Could you check a few things on this model? Use its own coordinates, in mm. Face numbers are marked on the shaded views. A direction names the side the tool comes from. Round coordinates to 2 decimals unless told otherwise and drop trailing zeros. Loops run counter-clockwise (first coordinate to the right, second up) from the corner with the lowest first, then second, coordinate; pieces in that order, holes last.
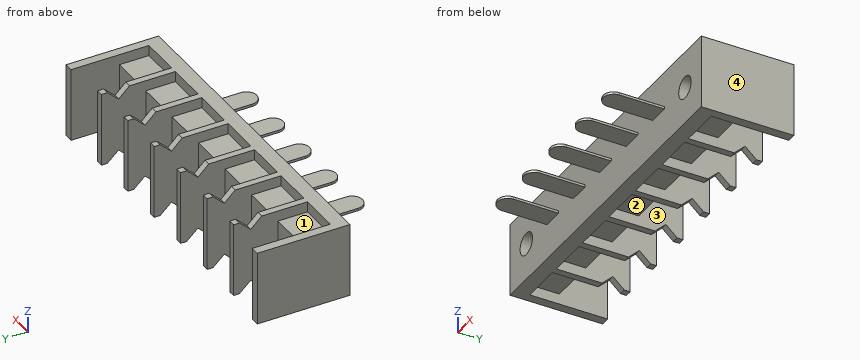
from build123d import *

# Parameters (mm, degrees)
SKETCH_1_W          = 69.1
SKETCH_1_H          = 15
EXTRUDE_1_DEPTH     = 18.8
SKETCH_2_W          = 65.5
SKETCH_2_H          = 15
CUT_EXTRUDE_1_DEPTH = 0.8
SKETCH_4_W          = 8.2
SKETCH_4_H          = 15
CUT_EXTRUDE_2_DEPTH = 9
SKETCH_5_W          = 8.2
SKETCH_5_H          = 2.132429546
CUT_EXTRUDE_3_DEPTH = 15
SKETCH_6_W          = 4.2
SKETCH_6_H          = 0.5
EXTRUDE_2_DEPTH     = 11.2
SKETCH_7_R          = 2.25
CUT_EXTRUDE_4_DEPTH = 41.718454047
CUT_EXTRUDE_START   = -49.1
CUT_EXTRUDE_5_DEPTH = 49.1
FILLET_1_R          = 2.1


with BuildPart() as part:
    # 草图1 → 拉伸1 (new body)
    with BuildSketch(Plane(origin=(0, 0, 0), x_dir=(1, 0, 0), z_dir=(0, 1, 0))):
        Rectangle(SKETCH_1_W, SKETCH_1_H)
    extrude(amount=EXTRUDE_1_DEPTH)

    # 草图2 → 切除-拉伸1 (cut)
    with BuildSketch(Plane(origin=(0, 18.8, 0), x_dir=(-1, 0, 0), z_dir=(0, 1, 0))):
        Rectangle(SKETCH_2_W, SKETCH_2_H)
    extrude(amount=-CUT_EXTRUDE_1_DEPTH, mode=Mode.SUBTRACT)

    # 草图4 → 切除-拉伸2 (cut)
    with BuildSketch(Plane(origin=(0, 18, 0), x_dir=(-1, 0, 0), z_dir=(0, 1, 0))):
        with Locations((-28.65, 0)):
            Rectangle(SKETCH_4_W, SKETCH_4_H)
        with Locations((-19.1, 0)):
            Rectangle(SKETCH_4_W, SKETCH_4_H)
        with Locations((-9.55, 0)):
            Rectangle(SKETCH_4_W, SKETCH_4_H)
        Rectangle(SKETCH_4_W, SKETCH_4_H)
        with Locations((9.55, 0)):
            Rectangle(SKETCH_4_W, SKETCH_4_H)
        with Locations((19.1, 0)):
            Rectangle(SKETCH_4_W, SKETCH_4_H)
        with Locations((28.65, 0)):
            Rectangle(SKETCH_4_W, SKETCH_4_H)
    extrude(amount=-CUT_EXTRUDE_2_DEPTH, mode=Mode.SUBTRACT)

    # 草图5 → 切除-拉伸3 (cut)
    with BuildSketch(Plane(origin=(0, 18, 0), x_dir=(-1, 0, 0), z_dir=(0, 1, 0))):
        with Locations((-28.65, -6.433785227)):
            Rectangle(SKETCH_5_W, SKETCH_5_H)
        with Locations((-28.65, 6.433785227)):
            Rectangle(SKETCH_5_W, SKETCH_5_H)
        with Locations((-19.1, -6.433785227)):
            Rectangle(SKETCH_5_W, SKETCH_5_H)
        with Locations((-19.1, 6.433785227)):
            Rectangle(SKETCH_5_W, SKETCH_5_H)
        with Locations((-9.55, -6.433785227)):
            Rectangle(SKETCH_5_W, SKETCH_5_H)
        with Locations((-9.55, 6.433785227)):
            Rectangle(SKETCH_5_W, SKETCH_5_H)
        with Locations((0, -6.433785227)):
            Rectangle(SKETCH_5_W, SKETCH_5_H)
        with Locations((0, 6.433785227)):
            Rectangle(SKETCH_5_W, SKETCH_5_H)
        with Locations((9.55, -6.433785227)):
            Rectangle(SKETCH_5_W, SKETCH_5_H)
        with Locations((9.55, 6.433785227)):
            Rectangle(SKETCH_5_W, SKETCH_5_H)
        with Locations((19.1, -6.433785227)):
            Rectangle(SKETCH_5_W, SKETCH_5_H)
        with Locations((19.1, 6.433785227)):
            Rectangle(SKETCH_5_W, SKETCH_5_H)
        with Locations((28.65, -6.433785227)):
            Rectangle(SKETCH_5_W, SKETCH_5_H)
        with Locations((28.65, 6.433785227)):
            Rectangle(SKETCH_5_W, SKETCH_5_H)
    extrude(amount=-CUT_EXTRUDE_3_DEPTH, mode=Mode.SUBTRACT)

    # 草图6 → 拉伸2 (add)
    with BuildSketch(Plane.XZ):
        Rectangle(SKETCH_6_W, SKETCH_6_H)
        with Locations((9.55, 0)):
            Rectangle(SKETCH_6_W, SKETCH_6_H)
        with Locations((19.1, 0)):
            Rectangle(SKETCH_6_W, SKETCH_6_H)
        with Locations((-9.55, 0)):
            Rectangle(SKETCH_6_W, SKETCH_6_H)
        with Locations((-19.1, 0)):
            Rectangle(SKETCH_6_W, SKETCH_6_H)
    extrude(amount=EXTRUDE_2_DEPTH)

    # 草图7 → 切除-拉伸4 (cut, through all)
    with BuildSketch(Plane(origin=(0, 9, 0), x_dir=(-1, 0, 0), z_dir=(0, 1, 0))):
        with Locations(Location((-28.65, 0, 0), (0, 0, 90))):
            Circle(SKETCH_7_R)
        with Locations(Location((28.65, 0, 0), (0, 0, 270))):
            Circle(SKETCH_7_R)
    extrude(amount=-CUT_EXTRUDE_4_DEPTH, mode=Mode.SUBTRACT)

    # 草图8 → 切除-拉伸5 (cut)
    with BuildSketch(Plane(origin=(24.55, 0, 0), x_dir=(0, 0, -1), z_dir=(1, 0, 0)).offset(CUT_EXTRUDE_START)):
        Polygon((7.5, 16.8), (5.4, 14.5), (7.5, 12.3), align=None)
        Polygon((-7.5, 16.8), (-7.5, 12.3), (-5.4, 14.5), align=None)
    extrude(amount=CUT_EXTRUDE_5_DEPTH, mode=Mode.SUBTRACT)

    # 圆角1
    fillet_1_edges = [part.edges().sort_by_distance(p)[0] for p in [
        (-21.2, -11.2, 0),
        (21.2, -11.2, 0),
        (17, -11.2, 0),
        (11.65, -11.2, 0),
        (7.45, -11.2, 0),
        (-2.1, -11.2, 0),
        (2.1, -11.2, 0),
        (-7.45, -11.2, 0),
        (-11.65, -11.2, 0),
        (-17, -11.2, 0),
    ]]
    fillet(fillet_1_edges, radius=FILLET_1_R - 0.0001)  # a hair under: the kernel refuses the full size


solid = part.part
Item 1: If we section it at D-D, the plane x = 16: Please give me the cut outline in (y, z), then the cut area to 3 significant figures.
Results list:
outline: (0, -7.5) - (3, -7.5) - (3, -5.37) - (9, -5.37) - (9, 5.37) - (3, 5.37) - (3, 7.5) - (0, 7.5) - close
area: 109 mm2
Item 2: For the marked faces 1 and 2, which set-ups out of +Z, -Z, +X, -X, +Y, -Y let a thin tool reach every point of the face, with its end or its side?
Results list:
face 1: +Z, +Y
face 2: -Z, +Y
Item 3: Will these pins go through, and if not, where does the flat tip stop? pin 1 (1.8 mm diameter, centred on x = -27.5, y = 7, fed in from -Z); pin 2 (0.6 mm diameter, centred on x = 28, z = -6, fed in from +Y); pin 3 (2.5 mm diameter, centred on x = -19.5, z = 6.5, fed in from +Y); pin 4 (8 mm diameter, centred on y = -5, z = -5, fed in from -X).
Results list:
pin 1: stops at z = -5.37
pin 2: stops at y = 3
pin 3: stops at y = 9
pin 4: passes through
Item 4: If we section it at A-A, the plane x = 28.65: Please give me the cut outline in (y, z).
Results list:
outline: (0, -7.5) - (3, -7.5) - (3, -5.37) - (9, -5.37) - (9, -2.25) - (0, -2.25) - close; (0, 2.25) - (9, 2.25) - (9, 5.37) - (3, 5.37) - (3, 7.5) - (0, 7.5) - close
Item 5: We'd pull the mould along X, two halves only. Please class the marked faces 3 and 4: released by +X, released by -X, zero draft, split by the parting line, or undercut.
Results list:
face 3: undercut
face 4: released by +X
Item 6: If I drill on line 1 along X through (y, z) = (5.25, 0); line 2 along Z through (x, y) = (-28.65, 4.75); line 3 along Y through (x, z) = (8, 4.5), over which ranges is the centre line in solid material (lowest first)?
Results list:
line 1: x = -34.55 to -30.9, -26.4 to 26.4, 30.9 to 34.55
line 2: z = -5.37 to -2.25, 2.25 to 5.37
line 3: y = 0 to 9
Item 7: If we section it at B-B, the plane y = -4.5: Please give me the cut outline in (x, z), then the cut area to 3 significant figures.
Results list:
outline: (-21.2, -0.25) - (-17, -0.25) - (-17, 0.25) - (-21.2, 0.25) - close; (-11.65, -0.25) - (-7.45, -0.25) - (-7.45, 0.25) - (-11.65, 0.25) - close; (-2.1, -0.25) - (2.1, -0.25) - (2.1, 0.25) - (-2.1, 0.25) - close; (7.45, -0.25) - (11.65, -0.25) - (11.65, 0.25) - (7.45, 0.25) - close; (17, -0.25) - (21.2, -0.25) - (21.2, 0.25) - (17, 0.25) - close
area: 10.5 mm2
